Autodesk Fusion 360 part; units mm, degrees
sketch "Sketch1" plane through (0, 0, 0) normal (0, 1, 0) x (1, 0, 0)
  line L0 (4.45, 0) -> (-4.45, 0)
  line L1 (-3.5, -8.6) -> (3.5, -8.6)
  line L2 (3.5, -8.6) -> (3.5, -6.6)
  line L3 (-3.5, -8.6) -> (-3.5, -6.6)
  line L4 (4.45, 0) -> (7.5, -3.05)
  line L5 (-4.45, 0) -> (-7.5, -3.05)
  line L6 (-4.45, 0) -> (-0.1366, 0) construction
  arc A0 (5.5, -6.6) -> (7.5, -3.05) centre (5.5, -4.2616) ccw
  arc A1 (-7.5, -3.05) -> (-5.5, -6.6) centre (-5.5, -4.2616) ccw
  line L7 (-5.5, -6.6) -> (-3.5, -6.6)
  line L8 (3.5, -6.6) -> (5.5, -6.6)
  dimension "d2" = 8.9
  dimension "d3" = 2
  dimension "d4" = 7
  dimension "d8" = 135
extrude "Extrude3" add sketch "Sketch1" along normal mid plane 20
sketch "Sketch2" plane through (0, 0, 8.6) normal (0, 0, 1) x (-1, 0, 0)
  line L0 (-3.5, 10) -> (-3.5, -10)
  line L1 (-3.5, -10) -> (3.5, -10)
  line L2 (3.5, -10) -> (3.5, 10)
  line L3 (3.5, 10) -> (-3.5, 10)
  circle A0 centre (0, 0) radius 2.5
  dimension "d22" = 5
extrude "Extrude4" cut sketch "Sketch2" against normal blind 8.8 contours A0
thread "Thread2"
fillet "Fillet4" radius 1 2 edges at (4.45, 0, 0) (-4.45, 0, 0)
fillet "Fillet5" radius 0.3 2 edges at (3.5, 0, 6.6) (-3.5, 0, 6.6)
fillet "Fillet6" radius 0.5 2 edges at (-3.5, 0, 8.6) (3.5, 0, 8.6)
Geometry: final body of the model. Coordinates: model frame, mm. A direction names the side the tool comes from. Give positions to 0.01 mm unless a question says otherwise; leave off trailing zeros. Loops run counter-clockwise (first coordinate to the right, second up) from the corner with the lowest first, then second, coordinate; pieces in that order, holes last. Notation, with made-up numbers: M 34,40 L 58,40 A24 cw 58,65 Z; hole C -10.75,55.25 d4. An arc over 180 degrees is marked long. Put each result on its own line as item: value. Start each with the question number.
1) Cut plane C-C (z = 1.25). Output: boundary loops of the cut face in (x, y), then the cut area to 3 significant figures.
2) Cut plane B-B (x = 0). Output: boundary loops of the cut face in (y, z), then the cut area to 3 significant figures.
3) Pull-direction query (X, two-part tool) for faces 4 (the flat face through (5, 0, 6.6)), 5 (the flat face through (-3.5, -0.1, 7.5)), 6 (the cylindrical face through (0.54, 2.44, 4.36)); classes: pulls with the +X half, pulls with the -X half, needs draft (parallel to the pull), parting line crosses it, or undercut.
4) Cut plane D-D (y = 2.75). Output: boundary loops of the cut face in (x, z).
5) Ray query, line 1 along Y through (x, z) = (0, 3.5); line 2 along Z through (x, y) = (-4, -2.5); line 3 along Y through (x, z) = (-1.5, 5.25). Return the intervals inside material, ascending.
6) Contact query for flat-ended pins moving along their axis: pin 1 (1 mm diameter, centred on y = -3.5, z = 7.5, fed in from -X); pin 2 (0.8 mm diameter, centred on x = 4.5, y = -0.5, fed in from +Z); pin 3 (1.3 mm diameter, centred on y = 1, z = 7.5, fed in from +X). Output: stop coordinate, or through.
7) Access query for faces 1 (the flat face through (3.5, -0.1, 7.5)), 2 (the flat face through (-5, 0, 6.6)), 3 (the flat face through (3, 0, 0)). Directions: +Z, -Z, +X, -X, +Y, -Y. A direction counts if a zero-diameter tool reaches every point of the face in a straight line with its end or side. Return the directions, or none.
8) Cut plane A-A (y = 0). Output: boundary loops of the cut face in (x, z), then the cut area to 3 significant figures.
Verdict:
1. outline: M -5.7,-10 L 5.7,-10 L 5.7,10 L -5.7,10 Z; hole C 0,0 d5
1. area: 208 mm2
2. outline: M -10,0 L -2.5,0 L -2.5,8.6 L -10,8.6 Z; M 2.5,0 L 10,0 L 10,8.6 L 2.5,8.6 Z
2. area: 129 mm2
3. face 4: needs draft
3. face 5: pulls with the -X half
3. face 6: undercut
4. outline: M -7.5,3.05 L -4.74,0.29 A1 ccw -4.04,0 L 4.04,0 A1 ccw 4.74,0.29 L 7.5,3.05 A2.34 ccw 5.5,6.6 L 3.8,6.6 A0.3 cw 3.5,6.9 L 3.5,8.1 A0.5 ccw 3,8.6 L -3,8.6 A0.5 ccw -3.5,8.1 L -3.5,6.9 A0.3 cw -3.8,6.6 L -5.5,6.6 A2.34 ccw Z
5. line 1: -10 to -2.5, 2.5 to 10
5. line 2: 0 to 6.6
5. line 3: -10 to -2, 2 to 10
6. pin 1: x = -3.5
6. pin 2: z = 6.6
6. pin 3: x = 3.5
7. face 1: +Z, +X, +Y, -Y
7. face 2: +Z, -X, +Y, -Y
7. face 3: -Z, +X, -X, +Y, -Y
8. outline: M -7.5,3.05 L -4.74,0.29 A1 ccw -4.04,0 L -2.5,0 L -2.5,8.6 L -3,8.6 A0.5 ccw -3.5,8.1 L -3.5,6.9 A0.3 cw -3.8,6.6 L -5.5,6.6 A2.34 ccw Z; M 2.5,0 L 4.04,0 A1 ccw 4.74,0.29 L 7.5,3.05 A2.34 ccw 5.5,6.6 L 3.8,6.6 A0.3 cw 3.5,6.9 L 3.5,8.1 A0.5 ccw 3,8.6 L 2.5,8.6 Z
8. area: 60.4 mm2
